Read the model definition and answer for the solid it produces. Units are mm, in the model's axes. Face numbers are marked on the shaded views. Coordinates: 2 decimals unless noted, no trailing zeros. Loops run counter-clockwise (first coordinate to the right, second up) from the corner with the lowest first, then second, coordinate; pieces in that order, holes last. Notation, with made-up numbers: M -32,-22.5 L -8,-22.5 A27 cw -8,6.5 Z; hole C -23.5,15 d1. An arc over 180 degrees is marked long. One line per item, written item: value. Start each with the question number.
1. The part is cut by section B-B (y = 0). Write down the section's boundary in (x, z), then the cut area to 3 significant figures.
2. Determine the mould class of the marked faces 1, 2 and 3 for opening direction Y: +Y half, -Y half, draft (parallel to the pull), parting line (faces both ways), or undercut.
3. The part is cut by section A-A (z = 58.1). Write down the section's boundary in (x, y).
4. Flat-ended cylindrical pins translate along their axes: pin 1 (2 mm diameter, centred on y = -7.78, z = 36.32, fed in from -X); pin 2 (1.5 mm diameter, centred on y = 6, z = 41, fed in from +X); pin 3 (1 mm diameter, centred on x = 0, z = 54, fed in from +Y). Find the tip coordinate at first contact, or state that the pin passes through.
5. The part is cut by section D-D (y = 11). Write down the section's boundary in (x, z), then the cut area to 3 significant figures.
6. The part is cut by section C-C (z = 44.1). Write down the section's boundary in (x, y), then the cut area to 3 significant figures.
7. Consider probe 1 along Y at (x, z) = (8, 73); probe 2 along Z at (x, y) = (-2, -7.5); probe 3 along X at (y, z) = (-10.5, 33.5). Determine where each line is inside the solid, lowest interval first.
```python
from build123d import *

# Parameters (mm, degrees)
BASE_FLANGE1_DEPTH = 88.2
CHAMFER1_SIZE      = 5
FILLET1_R          = 2.5
SKETCH4_R          = 5
CUT_EXTRUDE1_DEPTH = 92.368703613
SKETCH5_R          = 1.25
CUT_EXTRUDE2_DEPTH = 92.368703613
SKETCH6_R          = 1.25
CUT_EXTRUDE3_DEPTH = 98.361388651


# Sheet-metal steps are written as plain solids
with BuildPart() as part:
    # Sketch1 → Base-Flange1 (new body)
    with BuildSketch(Plane.XY):
        with BuildLine():
            Line((10, -17), (3, -17))
            ThreePointArc((3, -17), (0.878679656, -16.121320344), (0, -14))
            Line((0, -14), (0, 0))
            Line((0, 0), (0, 14))
            ThreePointArc((0, 14), (0.878679656, 16.121320344), (3, 17))
            Line((3, 17), (10, 17))
            Line((10, 17), (10, 20))
            Line((10, 20), (3, 20))
            ThreePointArc((3, 20), (-1.242640687, 18.242640687), (-3, 14))
            Line((-3, 14), (-3, 0))
            Line((-3, 0), (-3, -14))
            ThreePointArc((-3, -14), (-1.242640687, -18.242640687), (3, -20))
            Line((3, -20), (10, -20))
            Line((10, -20), (10, -17))
        make_face()
    extrude(amount=BASE_FLANGE1_DEPTH)

    # Chamfer1
    chamfer1_edges = [part.edges().sort_by_distance(p)[0] for p in [
        (10, 18.5, 0),
        (10, -18.5, 0),
        (10, 18.5, 88.2),
        (10, -18.5, 88.2),
    ]]
    chamfer(chamfer1_edges, length=CHAMFER1_SIZE)

    # Fillet1
    fillet1_edges = [part.edges().sort_by_distance(p)[0] for p in [
        (5, -18.5, 0),
        (10, -18.5, 83.2),
        (10, -18.5, 5),
        (5, 18.5, 0),
        (10, 18.5, 83.2),
        (10, 18.5, 5),
        (5, -18.5, 88.2),
        (5, 18.5, 88.2),
    ]]
    fillet(fillet1_edges, radius=FILLET1_R)

    # Sketch4 → Cut-Extrude1 (cut, through all)
    with BuildSketch(Plane.ZY.offset(3)):
        with Locations(Location((44.1, 0, 0), (0, 0, 270))):
            Circle(SKETCH4_R)
    extrude(amount=-CUT_EXTRUDE1_DEPTH, mode=Mode.SUBTRACT)

    # Sketch5 → Cut-Extrude2 (cut, through all)
    with BuildSketch(Plane.ZY.offset(3)):
        with Locations(Location((44.1, 11, 0), (0, 0, 270))):
            Circle(SKETCH5_R)
        with Locations(Location((51.878174593, 7.778174593, 0), (0, 0, 270))):
            Circle(SKETCH5_R)
        with Locations(Location((55.1, 0, 0), (0, 0, 270))):
            Circle(SKETCH5_R)
        with Locations(Location((51.878174593, -7.778174593, 0), (0, 0, 270))):
            Circle(SKETCH5_R)
        with Locations(Location((44.1, -11, 0), (0, 0, 270))):
            Circle(SKETCH5_R)
        with Locations(Location((36.321825407, -7.778174593, 0), (0, 0, 270))):
            Circle(SKETCH5_R)
        with Locations(Location((33.1, 0, 0), (0, 0, 270))):
            Circle(SKETCH5_R)
        with Locations(Location((36.321825407, 7.778174593, 0), (0, 0, 270))):
            Circle(SKETCH5_R)
    extrude(amount=-CUT_EXTRUDE2_DEPTH, mode=Mode.SUBTRACT)

    # Sketch6 → Cut-Extrude3 (cut, through all)
    with BuildSketch(Plane(origin=(0, 20, 0), x_dir=(1, 0, 0), z_dir=(0, 1, 0))):
        with Locations(Location((7.2, -79.1, 0), (0, 0, 270))):
            Circle(SKETCH6_R)
        with Locations(Location((7.2, -58.1, 0), (0, 0, 270))):
            Circle(SKETCH6_R)
        with Locations(Location((7.2, -30.1, 0), (0, 0, 90))):
            Circle(SKETCH6_R)
        with Locations(Location((7.2, -9.1, 0), (0, 0, 90))):
            Circle(SKETCH6_R)
    extrude(amount=-CUT_EXTRUDE3_DEPTH, mode=Mode.SUBTRACT)


solid = part.part
```
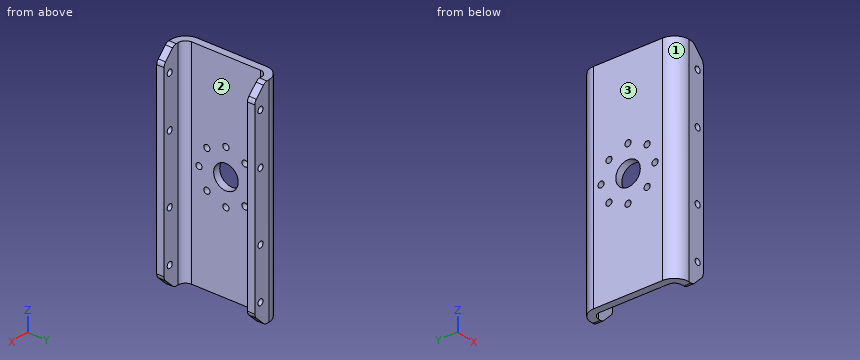
Answer block:
1. outline: M -3,0 L 0,0 L 0,31.85 L -3,31.85 Z; M -3,34.35 L 0,34.35 L 0,39.1 L -3,39.1 Z; M -3,49.1 L 0,49.1 L 0,53.85 L -3,53.85 Z; M -3,56.35 L 0,56.35 L 0,88.2 L -3,88.2 Z
1. area: 220 mm2
2. face 1: -Y half
2. face 2: undercut
2. face 3: draft
3. outline: M -3,-14 A6 ccw 3,-20 L 5.95,-20 L 5.95,-17 L 3,-17 A3 cw 0,-14 L 0,14 A3 cw 3,17 L 5.95,17 L 5.95,20 L 3,20 A6 ccw -3,14 Z; M 8.45,-20 L 10,-20 L 10,-17 L 8.45,-17 Z; M 8.45,17 L 10,17 L 10,20 L 8.45,20 Z
4. pin 1: passes through
4. pin 2: stops at x = 0
4. pin 3: stops at y = 19.45
5. outline: M -3,0 L 0,0 L 0,42.85 L -3,42.85 Z; M -3,45.35 L 0,45.35 L 0,88.2 L -3,88.2 Z
5. area: 257 mm2
6. outline: M -3,-14 A6 ccw 3,-20 L 10,-20 L 10,-17 L 3,-17 A3 cw 0,-14 L 0,-12.25 L -3,-12.25 Z; M -3,-9.75 L 0,-9.75 L 0,-5 L -3,-5 Z; M -3,5 L 0,5 L 0,9.75 L -3,9.75 Z; M -3,12.25 L 0,12.25 L 0,14 A3 cw 3,17 L 10,17 L 10,20 L 3,20 A6 ccw -3,14 Z
6. area: 123 mm2
7. probe 1: y = -20 to -17, 17 to 20
7. probe 2: z = 0 to 35.1, 37.54 to 50.66, 53.1 to 88.2
7. probe 3: x = -3 to 0
